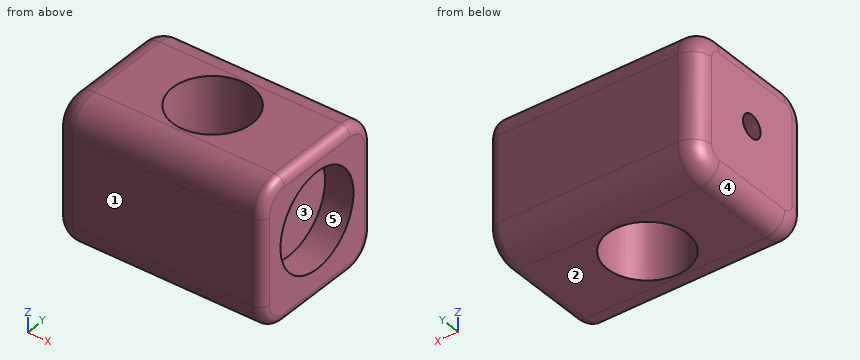
```python
from build123d import *

# Parameters (mm, degrees)
SKETCH_W        = 22
SKETCH_H        = 15
PAD_DEPTH       = 15
SKETCH001_R     = 4.2
POCKET_DEPTH    = 15.001
SKETCH002_R     = 5
POCKET001_DEPTH = 3
SKETCH003_R     = 1.2
POCKET002_DEPTH = 10
FILLET_R        = 3
FILLET001_R     = 1
FILLET002_R     = 2


with BuildPart() as part:
    # Sketch → Pad (new body)
    with BuildSketch(Plane.XY):
        Rectangle(SKETCH_W, SKETCH_H)
    extrude(amount=PAD_DEPTH)

    # Sketch001 → Pocket (cut, through all)
    with BuildSketch(Plane.XY.offset(15)):
        Circle(SKETCH001_R)
    extrude(amount=-POCKET_DEPTH, mode=Mode.SUBTRACT)

    # Sketch002 → Pocket001 (cut)
    with BuildSketch(Plane.YZ.offset(11)):
        with Locations((0, 8)):
            Circle(SKETCH002_R)
    extrude(amount=-POCKET001_DEPTH, mode=Mode.SUBTRACT)

    # Sketch003 → Pocket002 (cut)
    with BuildSketch(Plane(origin=(-11, 0, 0), x_dir=(0, -1, 0), z_dir=(-1, 0, 0))):
        with Locations((0, 8)):
            Circle(SKETCH003_R)
    extrude(amount=-POCKET002_DEPTH, mode=Mode.SUBTRACT)

    # Fillet
    fillet_edges = [part.edges().sort_by_distance(p)[0] for p in [
        (0, -7.5, 15),
        (0, -7.5, 0),
        (0, 7.5, 15),
        (0, 7.5, 0),
    ]]
    fillet(fillet_edges, radius=FILLET_R)

    # Fillet001
    fillet001_edges = [part.edges().sort_by_distance(p)[0] for p in [
        (11, 0, 15),
    ]]
    fillet(fillet001_edges, radius=FILLET001_R)

    # Fillet002
    fillet002_edges = [part.edges().sort_by_distance(p)[0] for p in [
        (-11, 0, 0),
    ]]
    fillet(fillet002_edges, radius=FILLET002_R)


solid = part.part
```
Work out the finished part from the listing and answer in its coordinate system (mm). Face numbers are marked on the shaded views. A direction names the side the tool comes from. Coordinates: 2 decimals unless noted, no trailing zeros. Loops run counter-clockwise (first coordinate to the right, second up) from the corner with the lowest first, then second, coordinate; pieces in that order, holes last. Notation, with made-up numbers: M 10,-7.75 L 51,-7.75 A17 ccw 51,3.25 Z; hole C -21.5,72 d6. An arc over 180 degrees is marked long. Use CSV: the item, a comma, the result in double quotes. Start each with the question number.
(1) For the marked faces 4 and 5, determine the directions among +Z, -Z, +X, -X, +Y, -Y from which every point of the face is accessible in a straight line to the end or side of a thin tool.
(2) Given pin 1 Ø8 at (y, z) = (-2.5, 9.5) entering from +X; pin 2 Ø6.5 at (x, y) = (0, 0) entering from -Z; pin 3 Ø1.9 at (y, z) = (0, 8) entering from +X, each flat-ended and moving along its own axis, determine where each tip first touches the part or whether it passes through.
(3) Find section B-B, the plane y = 0. Give the vertices of the cut face in (x, z).
(4) For a pull along Y with two mould halves and no side action, classify the marked faces 1, 2 and 3 as +Y half, -Y half, draft (parallel to the pull), parting line (faces both ways), or undercut.
(5) Find section A-A, the plane x = 0. Give the vertices of the cut face in (y, z), then the cut area to 3 significant figures.
(6) Consider line 1 (Z direction, x = 9.9, y = 0); line 2 (Y direction, x = 0, z = 9.25); line 3 (Y direction, x = -9, z = 8). Determine where each line is inside the solid, lowest interval first.
(7) Find section C-C, the plane z = 8. Give the vertices of the cut face in (x, y), then the cut area to 3 significant figures.
(8) Find section D-D, the plane x = 8.5. Give the vertices of the cut face in (y, z), then the cut area to 3 significant figures.
Recorded:
1,face 4,"-Z, -X, +Y, -Y"
1,face 5,"+X"
2,pin 1,"stops at x = 11"
2,pin 2,"passes through"
2,pin 3,"stops at x = 8"
3,outline,"M -11,2 A2 ccw -9,0 L -4.2,0 L -4.2,6.8 L -11,6.8 Z; M -11,9.2 L -4.2,9.2 L -4.2,15 L -9,15 A2 ccw -11,13 Z; M 4.2,0 L 10,0 A1 ccw 11,1 L 11,3 L 8,3 L 8,13 L 11,13 L 11,14 A1 ccw 10,15 L 4.2,15 Z"
4,face 1,"-Y half"
4,face 2,"draft"
4,face 3,"undercut"
5,outline,"M -7.5,3 A3 ccw -4.5,0 L -4.2,0 L -4.2,15 L -4.5,15 A3 ccw -7.5,12 Z; M 4.2,0 L 4.5,0 A3 ccw 7.5,3 L 7.5,12 A3 ccw 4.5,15 L 4.2,15 Z"
5,area,"91.3 mm^2"
6,line 1,"z = 0 to 3, 13 to 15"
6,line 2,"y = -7.5 to -4.2, 4.2 to 7.5"
6,line 3,"y = -7.5 to -1.2, 1.2 to 7.5"
7,outline,"M -11,-5.5 A2 ccw -9,-7.5 L 10,-7.5 A1 ccw 11,-6.5 L 11,-5 L 8,-5 L 8,5 L 11,5 L 11,6.5 A1 ccw 10,7.5 L -9,7.5 A2 ccw -11,5.5 L -11,1.2 L -4.02,1.2 A4.2 cw long -4.02,-1.2 L -11,-1.2 Z"
7,area,"226 mm^2"
8,outline,"M -7.5,3 A3 ccw -4.5,0 L 4.5,0 A3 ccw 7.5,3 L 7.5,12 A3 ccw 4.5,15 L -4.5,15 A3 ccw -7.5,12 Z; hole C 0,8 d10"
8,area,"139 mm^2"
